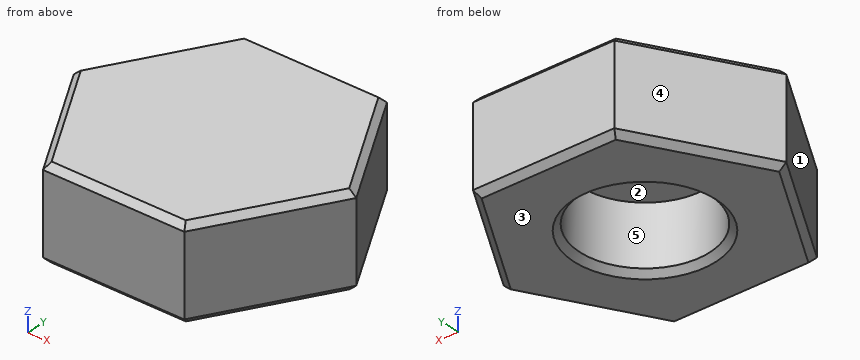
from build123d import *

# Parameters (mm, degrees)
PAD_DEPTH       = 3
SKETCH001_R     = 2.125
POCKET_DEPTH    = 2.15
CHAMFER_SIZE    = 0.2
CHAMFER001_SIZE = 0.2


with BuildPart() as part:
    # Sketch → Pad (new body)
    with BuildSketch(Plane.XY):
        Polygon((4.618802, 0), (2.309401, 4), (-2.309401, 4), (-4.618802, 0), (-2.309401, -4), (2.309401, -4), align=None)
    extrude(amount=PAD_DEPTH)

    # Sketch001 → Pocket (cut)
    with BuildSketch(Plane.XY):
        Circle(SKETCH001_R)
    extrude(amount=POCKET_DEPTH, mode=Mode.SUBTRACT)

    # Chamfer
    chamfer_edges = [part.edges().sort_by_distance(p)[0] for p in [
        (3.464102, 2, 3),
        (0, 4, 3),
        (-3.464102, 2, 3),
        (-3.464102, -2, 3),
        (0, -4, 3),
        (3.464102, -2, 3),
    ]]
    chamfer(chamfer_edges, length=CHAMFER_SIZE)

    # Chamfer001
    chamfer001_edges = [part.edges().sort_by_distance(p)[0] for p in [
        (3.464102, 2, 0),
        (3.464102, -2, 0),
        (0, 4, 0),
        (0, -4, 0),
        (-3.464102, 2, 0),
        (-3.464102, -2, 0),
        (-2.125, 0, 0),
    ]]
    chamfer(chamfer001_edges, length=CHAMFER001_SIZE)


solid = part.part
Design review of the part built by this model. Coordinates are the model's own, in mm. Face numbers are marked on the shaded views. A direction names the side the tool comes from. Round coordinates to 2 decimals unless told otherwise and drop trailing zeros. Loops run counter-clockwise (first coordinate to the right, second up) from the corner with the lowest first, then second, coordinate; pieces in that order, holes last. Notation, with made-up numbers: M 36.25,43 L 49.25,43 A25 cw 49.25,66 Z; hole C 47.5,79.5 d1. An arc over 180 degrees is marked long. Answer as a JSON object with one key per item and string values.
Item 1: Clearance check with flat-ended pins moving along their axes: P1, Ø1.5, axis at y = 3, z = 0.5, coming from the -X side; P2, Ø1.3, axis at x = -1, y = 0, coming from the -Z side. State where each tip first meets the part, or that it passes through.
Answer sheet:
{"P1": "stops at x = -3.32", "P2": "stops at z = 2.15"}
Item 2: We need section A-A on z = 0.95. Give the boundary of the cut face in (x, y) (3 decimals), and give its area (3 significant figures).
Answer sheet:
{"outline": "M -4.619,0 L -2.309,-4 L 2.309,-4 L 4.619,0 L 2.309,4 L -2.309,4 Z; hole C 0,0 d4.25", "area": "41.2 mm^2"}
Item 3: We need section B-B on x = 0. Give the boundary of the cut face in (y, z) (3 decimals).
Answer sheet:
{"outline": "M -4,0.2 L -3.8,0 L -2.325,0 L -2.125,0.2 L -2.125,2.15 L 2.125,2.15 L 2.125,0.2 L 2.325,0 L 3.8,0 L 4,0.2 L 4,2.8 L 3.8,3 L -3.8,3 L -4,2.8 Z"}
Item 4: We need section D-D on y = -3.5. Give the boundary of the cut face in (x, z).
Answer sheet:
{"outline": "M -2.6,0.2 L -2.37,0 L 2.37,0 L 2.6,0.2 L 2.6,2.8 L 2.37,3 L -2.37,3 L -2.6,2.8 Z"}
Item 5: We need section C-C on z = 2.65. Give the boundary of the cut face in (x, y).
Answer sheet:
{"outline": "M -4.62,0 L -2.31,-4 L 2.31,-4 L 4.62,0 L 2.31,4 L -2.31,4 Z"}
Item 6: The part is to be moulded in two halves that separate along Y. For the marked faces 1, 2 and 3, say which applies: pulls with the +Y half, pulls with the -Y half, needs draft (parallel to the pull), parting line crosses it, or undercut.
Answer sheet:
{"face 1": "pulls with the -Y half", "face 2": "undercut", "face 3": "needs draft"}
Item 7: Machinability: for the marked faces 4 and 5, which of the approach directions +Z, -Z, +X, -X, +Y, -Y give a long, thin tool a straight path to every point of the face, cutting with its end or side? Answer none if there is none.
Answer sheet:
{"face 4": "+Z, -Z, -X, +Y", "face 5": "-Z"}
Item 8: Wall thickness on L1, parallel to Y at x = 0, z = 1.4 (3 decimals); L2, parallel to Y at x = -1.75, z = 1.1; L3, parallel to Z at x = -1.25, y = 1.25: over which ranges is each line inside the solid? List them lowest first. Write a range as from..to.
Answer sheet:
{"L1": "y = -4..-2.125, 2.125..4", "L2": "y = -4..-1.21, 1.21..4", "L3": "z = 2.15..3"}
